Part model, mm, in its own coordinate system. A direction names the side the tool comes from. Round coordinates to 2 decimals unless told otherwise and drop trailing zeros. Write each loop counter-clockwise with the first axis right and the second up, starting at its lowest first coordinate (ties: lowest second). Pieces come first, ordered by that corner, then holes. Notation, with made-up numbers: (54, 31) -> (73, 31) arc R33 ccw to (73, 66) -> close; hole circle Ø7 at (2, -13). An arc over 180 degrees is marked (long way). Return JSON: item names as keys, results as strings. Group by question number.
Autodesk Inventor part; units mm, degrees
ref_plane "YZ Plane" through (0, 0, 0) normal (1, 0, 0) x (0, 1, 0)
ref_plane "XZ Plane" through (0, 0, 0) normal (0, 1, 0) x (-1, 0, 0)
ref_plane "XY Plane" through (0, 0, 0) normal (0, 0, 1) x (1, 0, 0)
sketch "Skizze2" plane through (0, 0, 0) normal (0, 0, 1) x (1, 0, 0)
  line L0 (2.4, 0) -> (2.4, 7)
  line L1 (-2.4, 0) -> (-2.4, 7)
  line L2 (0, 0) -> (2.4, 0) construction
  line L3 (-2.4, 7) -> (2.4, 7)
  line L4 (-2.4, 0) -> (-4.6, 0)
  line L5 (2.4, 0) -> (4.6, 0)
  arc A0 (-4.6, 0) -> (4.6, 0) centre (0, 4.29) ccw
  point P0 (0, -2)
  dimension "d0" = 7
  dimension "d1" = 4.8
  dimension "d2" = 2.4
  dimension "d3" = 2.2
  dimension "d4" = 2
extrude "Extrusion1" add sketch "Skizze2" along normal blind 5
sketch "Skizze3" plane through (0, 0, 5) normal (0, 0, 1) x (1, 0, 0)
  line L0 (-2.4, 0) -> (-2.4, 2.2) construction
  line L1 (-2.4, 2.2) -> (-10, 2.2)
  line L2 (-2.4, 2.2) -> (10, 2.2)
  line L3 (-10, 2.2) -> (10, 2.2)
  line L4 (10, 2.2) -> (10, 7)
  line L5 (10, 7) -> (-10, 7)
  line L6 (-10, 7) -> (-10, 2.2)
  point P0 (0, 0)
  point P1 (2.4, 7)
  dimension "d7" = 2.2
  dimension "d8" = 20
  dimension "d9" = 10
  dimension "d10" = 20
extrude "Extrusion2" add sketch "Skizze3" against normal blind 5
sketch "Skizze5" plane through (-10, 2.2, 5) normal (-1, 0, 0) x (0, 0, 1)
  line L0 (0, 4.8) -> (-5, 4.8)
  line L1 (-5, 4.8) -> (0, 4.8)
  line L2 (0, 4.8) -> (0, -0.0545)
  line L3 (0, -0.0545) -> (-5, -0.0545)
  line L4 (-5, -0.0545) -> (-5, 4.8)
  point P0 (-5, -2.2)
extrude "Extrusion3" add sketch "Skizze5" along normal blind 5
sketch "Skizze6" plane through (-10, 2.1455, 0) normal (0, -1, 0) x (1, 0, 0)
  line L0 (0, 5) -> (7.6, 5)
  line L1 (0, 5) -> (-5, 5)
  line L2 (0, 5) -> (-5, 5)
  line L3 (-5, 5) -> (-5, 0)
  line L4 (-5, 0) -> (0, 0)
  line L5 (0, 0) -> (0, 5)
  point P0 (10, 0)
extrude "Extrusion4" add sketch "Skizze6" against normal blind 25
sketch "Skizze12" plane through (-15, 2.2, 5) normal (-1, 0, 0) x (0, 0, 1)
  line L0 (0, -0.0545) -> (0, 24.9455)
  line L1 (-5, -0.0545) -> (-5, 24.9455)
  line L2 (0, -0.0545) -> (-5, -0.0545)
  line L3 (-5, -0.0545) -> (-5, 24.9455)
  line L4 (-5, 24.9455) -> (0, 24.9455)
  line L5 (0, 24.9455) -> (0, -0.0545)
  point P0 (-5, -2.2)
extrude "Extrusion9" add sketch "Skizze12" along normal blind 15
sketch "Skizze13" plane through (0, 0, 5) normal (0, 0, 1) x (1, 0, 0)
  circle A0 centre (-20, 17.1455) radius 7.5
  line L0 (-10, 27.1455) -> (-30, 27.1455)
  line L1 (-30, 2.1455) -> (-30, 27.1455)
  point P0 (0, 0)
  point P1 (-20, 27.1455)
  dimension "d31" = 15
  dimension "d32" = 10
  dimension "d33" = 10
extrude "Extrusion10" cut sketch "Skizze13" against normal blind 15
sketch "Skizze14" plane through (0, 0, 0) normal (0, 0, -1) x (-1, 0, 0)
  line L0 (10, 2.2) -> (10, 2.1455)
  line L1 (10, 2.2) -> (10, 2.1455)
  line L2 (10, 2.1455) -> (-9.9939, 2.1455)
  line L3 (-10, 2.2) -> (-2.4, 2.2)
  line L4 (-9.9939, 2.1455) -> (-10, 2.2)
  line L5 (-10, 2.2) -> (10, 2.2)
  point P0 (0, 0)
extrude "Extrusion11" add sketch "Skizze14" against normal blind 5
sketch "Skizze16" plane through (0, 0, 0) normal (0, 0, -1) x (-1, 0, 0)
  line L0 (2.4, 2.1455) -> (30, 2.1455)
  line L1 (30, 27.1455) -> (30, 2.1455)
  line L2 (10, 27.1455) -> (30, 27.1455)
  line L3 (10, 7) -> (10, 27.1455)
  line L4 (-10, 7) -> (10, 7)
  line L5 (-10, 7) -> (-10, 2.2)
  line L6 (-10, 2.2) -> (-9.9939, 2.1455)
  line L7 (-9.9939, 2.1455) -> (-2.4, 2.1455)
  line L8 (-2.4, 0) -> (-2.4, 2.1455)
  line L9 (-4.6, 0) -> (-2.4, 0)
  arc A0 (-4.6, 0) -> (4.6, 0) centre (0, 4.29) ccw
  line L10 (2.4, 0) -> (4.6, 0)
  line L11 (2.4, 2.1455) -> (2.4, 0)
  circle A1 centre (20, 17.1455) radius 7.5
  point P0 (0, 0)
extrude "Extrusion12" add sketch "Skizze16" along normal blind 17.8
sketch "Skizze17" plane through (-10, 27.1455, 0) normal (0, 1, 0) x (1, 0, 0)
  line L0 (0, -5) -> (-20, -5)
  line L1 (0, -5) -> (0, 17.8)
  line L2 (-20, 17.8) -> (0, 17.8)
  line L3 (-20, -5) -> (-20, 17.8)
  line L4 (0, 7.8) -> (-20, 7.8)
  line L5 (-20, -5) -> (-20, 17.8)
  line L6 (-20, 7.8) -> (-20, 0)
  line L7 (-20, 0) -> (0, 0)
  line L8 (0, 7.8) -> (0, 0)
  point P0 (10, 0)
  dimension "d41" = 10
  dimension "d42" = 7.8
extrude "Extrusion13" cut sketch "Skizze17" against normal through all contours L7 L3 L4 L1
fillet "Rundung3" radius 2 2 edges at (-27.5, 17.1455, 5) (-12.5, 17.1455, -17.8)
properties part number "Connector MiniTec"
Item 1: Wall check: L1, parallel to Y at x = -20, z = -12.25; L2, parallel to Z at x = -25, y = 6.25; L3, parallel to X at y = 22.25, z = -8. Give the ranges that are in metal, low to high.
Item 2: Two-plate mould, pull along X, no slides. Class faces 1 (the face through (-27.493, 17.475, 1.521)), 2 (the face through (-10, 17, -13)), 3 (the face through (-30, 15, -13)): released by +X, released by -X, zero draft, split by the parting line, or undercut.
Item 3: Flat gauge pins, fed straight in: P1, Ø1.1, axis at y = 1.5, z = -2, coming from the -X side; P2, Ø2.5, axis at x = 7, z = -5, coming from the -Y side; P3, Ø1, axis at y = 1.5, z = 0, coming from the +X side. Where does each tip first touch, or does it go through?
Item 4: Cut at B-B (z = -4). Write the cut outline in (x, y), then the cut area to 3 significant figures.
Item 5: Which spindle directions (+Z, -Z, +X, -X, +Y, -Y) get a long thin tool onto all of the face, cutting with end or side? Do faces 4 (the face through (6, 2.146, -6)), 5 (the face through (-10, 5, -4)), 6 (the face through (-2.4, 1, -6)). Say none if no direction does.
Item 6: Cut at D-D (z = -14.5). Write the cut outline in (x, y), then the cut area to 3 significant figures.
Item 7: Cut at A-A (x = -20). Write the cut outline in (y, z).
Item 8: Cut at C-C (y = 5.5). Write the cut outline in (x, z).
Checks:
{
 "1": {"L1": "y = 2.15 to 9.65, 24.65 to 27.15", "L2": "z = -17.8 to -7.8, 0 to 5", "L3": "x = -30 to -25.49, -14.51 to -10"},
 "2": {"face 1": "undercut", "face 2": "released by +X", "face 3": "released by -X"},
 "3": {"P1": "stops at x = -2.4", "P2": "stops at y = 2.15", "P3": "stops at x = 2.4"},
 "4": {"outline": "(-10, 2.15) -> (-2.4, 2.15) -> (-2.4, 0) -> (-4.6, 0) arc R6.29 ccw to (4.6, 0) -> (2.4, 0) -> (2.4, 2.15) -> (9.99, 2.15) -> (10, 2.2) -> (10, 7) -> (-10, 7) -> close", "area": "120 mm2"},
 "5": {"face 4": "+Z, -Z, +X", "face 5": "-X, +Y, -Y", "face 6": "+Z, -Z, -X"},
 "6": {"outline": "(-30, 2.15) -> (-2.4, 2.15) -> (-2.4, 0) -> (-4.6, 0) arc R6.29 ccw to (4.6, 0) -> (2.4, 0) -> (2.4, 2.15) -> (9.99, 2.15) -> (10, 2.2) -> (10, 7) -> (-10, 7) -> (-10, 27.15) -> (-30, 27.15) -> close; hole circle Ø15 at (-20, 17.15)", "area": "443 mm2"},
 "7": {"outline": "(2.15, -17.8) -> (7.65, -17.8) arc R2 ccw to (9.65, -15.8) -> (9.65, -7.8) -> (2.15, -7.8) -> close; (2.15, 0) -> (9.65, 0) -> (9.65, 3) arc R2 ccw to (7.65, 5) -> (2.15, 5) -> close; (24.65, -15.8) arc R2 ccw to (26.65, -17.8) -> (27.15, -17.8) -> (27.15, -7.8) -> (24.65, -7.8) -> close; (24.65, 0) -> (27.15, 0) -> (27.15, 5) -> (26.65, 5) arc R2 ccw to (24.65, 3) -> close"},
 "8": {"outline": "(-30, -17.8) -> (10, -17.8) -> (10, 5) -> (-30, 5) -> (-30, 0) -> (-10, 0) -> (-10, -7.8) -> (-30, -7.8) -> close"}
}
